```python
from build123d import *

# Parameters (mm, degrees)
SKETCH2_R           = 1.6
BOSS_EXTRUDE1_DEPTH = 4
CUT_EXTRUDE1_DEPTH  = 2
CUT_EXTRUDE2_DEPTH  = 1.5
SKETCH5_R           = 1.5
CUT_EXTRUDE3_DEPTH  = 52.039200621
BOSS_EXTRUDE2_START = 1.5
SKETCH6_R           = 4
SKETCH6_R_2         = 1.5
BOSS_EXTRUDE2_DEPTH = 1.5
CIRPATTERN1_COUNT   = 4
FILLET1_R           = 1
FILLET2_R           = 30


with BuildPart() as part:
    # Sketch2 → Boss-Extrude1 (new body)
    with BuildSketch(Plane(origin=(0, 0, 0), x_dir=(1, 0, 0), z_dir=(0, 1, 0))):
        Polygon((-12.5, 35), (12.5, 35), (23.334523779, 36.062445841), (36.062445841, 23.334523779), (35, 12.5), (35, -12.5), (36.062445841, -23.334523779), (23.334523779, -36.062445841), (12.5, -35), (-12.5, -35), (-23.334523779, -36.062445841), (-36.062445841, -23.334523779), (-35, -12.5), (-35, 12.5), (-36.062445841, 23.334523779), (-23.334523779, 36.062445841), align=None)
        with Locations(Location((22.627416998, 31.112698372, 0), (0, 0, 270))):
            Circle(SKETCH2_R, mode=Mode.SUBTRACT)
        with Locations(Location((31.112698372, 22.627416998, 0), (0, 0, 270))):
            Circle(SKETCH2_R, mode=Mode.SUBTRACT)
        with Locations(Location((22.627416998, -31.112698372, 0), (0, 0, 270))):
            Circle(SKETCH2_R, mode=Mode.SUBTRACT)
        with Locations(Location((31.112698372, -22.627416998, 0), (0, 0, 270))):
            Circle(SKETCH2_R, mode=Mode.SUBTRACT)
        with Locations(Location((-31.112698372, -22.627416998, 0), (0, 0, 270))):
            Circle(SKETCH2_R, mode=Mode.SUBTRACT)
        with Locations(Location((-22.627416998, -31.112698372, 0), (0, 0, 270))):
            Circle(SKETCH2_R, mode=Mode.SUBTRACT)
        with Locations(Location((-22.627416998, 31.112698372, 0), (0, 0, 270))):
            Circle(SKETCH2_R, mode=Mode.SUBTRACT)
        with Locations(Location((-31.112698372, 22.627416998, 0), (0, 0, 270))):
            Circle(SKETCH2_R, mode=Mode.SUBTRACT)
    extrude(amount=BOSS_EXTRUDE1_DEPTH)

    # Sketch3 → Cut-Extrude1 (cut)
    with BuildSketch(Plane(origin=(0, 4, 0), x_dir=(1, 0, 0), z_dir=(0, 1, 0))):
        Polygon((-17.669047558, 29), (17.669047558, 29), (29, 17.669047558), (29, -17.669047558), (17.669047558, -29), (-17.669047558, -29), (-29, -17.669047558), (-29, 17.669047558), align=None)
    extrude(amount=-CUT_EXTRUDE1_DEPTH, mode=Mode.SUBTRACT)

    # Sketch4 → Cut-Extrude2 (cut)
    with BuildSketch(Plane(origin=(0, 2, 0), x_dir=(1, 0, 0), z_dir=(0, 1, 0))):
        with BuildLine():
            Line((-29, 11.263085893), (-29, -11.263085893))
            ThreePointArc((-29, -11.263085893), (-27.272329864, -13.979918004), (-24.079215521, -13.567556979))
            Line((-24.079215521, -13.567556979), (-16.079215521, -6.899529803))
            ThreePointArc((-16.079215521, -6.899529803), (-15.283167889, -5.867388581), (-15, -4.595058717))
            Line((-15, -4.595058717), (-15, 4.595058717))
            ThreePointArc((-15, 4.595058717), (-15.283167889, 5.867388581), (-16.079215521, 6.899529803))
            Line((-16.079215521, 6.899529803), (-24.079215521, 13.567556979))
            ThreePointArc((-24.079215521, 13.567556979), (-27.272329864, 13.979918004), (-29, 11.263085893))
        make_face()
        with BuildLine():
            Line((11.263085893, 29), (-11.263085893, 29))
            ThreePointArc((-11.263085893, 29), (-13.979918004, 27.272329864), (-13.567556979, 24.079215521))
            Line((-13.567556979, 24.079215521), (-6.899529803, 16.079215521))
            ThreePointArc((-6.899529803, 16.079215521), (-5.867388581, 15.283167889), (-4.595058717, 15))
            Line((-4.595058717, 15), (4.595058717, 15))
            ThreePointArc((4.595058717, 15), (5.867388581, 15.283167889), (6.899529803, 16.079215521))
            Line((6.899529803, 16.079215521), (13.567556979, 24.079215521))
            ThreePointArc((13.567556979, 24.079215521), (13.979918004, 27.272329864), (11.263085893, 29))
        make_face()
        with BuildLine():
            Line((29, -11.263085893), (29, 11.263085893))
            ThreePointArc((29, 11.263085893), (27.272329864, 13.979918004), (24.079215521, 13.567556979))
            Line((24.079215521, 13.567556979), (16.079215521, 6.899529803))
            ThreePointArc((16.079215521, 6.899529803), (15.283167889, 5.867388581), (15, 4.595058717))
            Line((15, 4.595058717), (15, -4.595058717))
            ThreePointArc((15, -4.595058717), (15.283167889, -5.867388581), (16.079215521, -6.899529803))
            Line((16.079215521, -6.899529803), (24.079215521, -13.567556979))
            ThreePointArc((24.079215521, -13.567556979), (27.272329864, -13.979918004), (29, -11.263085893))
        make_face()
        with BuildLine():
            Line((-11.263085893, -29), (11.263085893, -29))
            ThreePointArc((11.263085893, -29), (13.979918004, -27.272329864), (13.567556979, -24.079215521))
            Line((13.567556979, -24.079215521), (6.899529803, -16.079215521))
            ThreePointArc((6.899529803, -16.079215521), (5.867388581, -15.283167889), (4.595058717, -15))
            Line((4.595058717, -15), (-4.595058717, -15))
            ThreePointArc((-4.595058717, -15), (-5.867388581, -15.283167889), (-6.899529803, -16.079215521))
            Line((-6.899529803, -16.079215521), (-13.567556979, -24.079215521))
            ThreePointArc((-13.567556979, -24.079215521), (-13.979918004, -27.272329864), (-11.263085893, -29))
        make_face()
    extrude(amount=-CUT_EXTRUDE2_DEPTH, mode=Mode.SUBTRACT)

    # Sketch5 → Cut-Extrude3 (cut, through all)
    with BuildSketch(Plane(origin=(0, 2, 0), x_dir=(1, 0, 0), z_dir=(0, 1, 0))):
        with Locations(Location((13.22775948, 15.25, 0), (0, 0, 270))):
            Circle(SKETCH5_R)
    cut_extrude3 = extrude(amount=-CUT_EXTRUDE3_DEPTH, mode=Mode.SUBTRACT)

    # Sketch6 → Boss-Extrude2 (add)
    with BuildSketch(Plane(origin=(0, 2, 0), x_dir=(1, 0, 0), z_dir=(0, 1, 0)).offset(BOSS_EXTRUDE2_START)):
        with Locations(Location((13.22775948, 15.25, 0), (0, 0, 90))):
            Circle(SKETCH6_R)
        with Locations(Location((13.22775948, 15.25, 0), (0, 0, 270))):
            Circle(SKETCH6_R_2, mode=Mode.SUBTRACT)
    boss_extrude2 = extrude(amount=-BOSS_EXTRUDE2_DEPTH)

    # CirPattern1: Cut-Extrude3, Boss-Extrude2 ×4 about axis
    cirpattern1_axis = Axis((0, 0, 0), (0, 1, 0))
    add([cut_extrude3.rotate(cirpattern1_axis, i * 360 / CIRPATTERN1_COUNT) for i in range(1, CIRPATTERN1_COUNT)], mode=Mode.SUBTRACT)
    add([boss_extrude2.rotate(cirpattern1_axis, i * 360 / CIRPATTERN1_COUNT) for i in range(1, CIRPATTERN1_COUNT)])

    # Fillet1
    fillet1_edges = [part.edges().sort_by_distance(p)[0] for p in [
        (13.22775948, 2, -11.25),
        (-11.25, 2, -13.22775948),
        (-13.22775948, 2, 11.25),
        (11.25, 2, 13.22775948),
    ]]
    fillet(fillet1_edges, radius=FILLET1_R)

    # Fillet2
    # the kernel refuses this fillet: 30 mm, written as the material it adds along each edge
    with BuildSketch(Plane(origin=(-12.5, 0, -35), x_dir=(1, 0, 0), z_dir=(0, 1, 0)), Plane(origin=(-12.5, 0, 35), x_dir=(-0.9952264052892463, 0, 0.09759304388656388), z_dir=(0, 1, 0)), Plane(origin=(-35, 0, 12.5), x_dir=(0, 0, -1), z_dir=(0, 1, 0)), Plane(origin=(-35, 0, -12.5), x_dir=(-0.09759304388655968, 0, -0.9952264052892468), z_dir=(0, 1, 0))) as fillet2_piece_1:
        with BuildLine():
            CenterArc((FILLET2_R * 0.0489132680018, FILLET2_R), FILLET2_R, 264.399415997, 5.600584003)
            Line((-FILLET2_R * 0.0486797758844, FILLET2_R * 0.00477359471072), (0, 0))
            Line((0, 0), (FILLET2_R * 0.0489132680018, 0))
        make_face()
    extrude(amount=4)
    with BuildSketch(Plane(origin=(12.5, 0, -35), x_dir=(-1, 0, 0), z_dir=(0, 1, 0)), Plane(origin=(35, 0, -12.5), x_dir=(0.09759304388620155, 0, -0.9952264052892819), z_dir=(0, 1, 0)), Plane(origin=(35, 0, 12.5), x_dir=(0, 0, -1), z_dir=(0, 1, 0)), Plane(origin=(12.5, 0, 35), x_dir=(0.9952264052892817, 0, 0.09759304388620309), z_dir=(0, 1, 0))) as fillet2_piece_2:
        with BuildLine():
            CenterArc((FILLET2_R * 0.048913268002, -FILLET2_R), FILLET2_R, 90, 5.600584003)
            Line((-FILLET2_R * 0.0486797758846, -FILLET2_R * 0.00477359471075), (0, 0))
            Line((0, 0), (FILLET2_R * 0.048913268002, 0))
        make_face()
    extrude(amount=4)


solid = part.part
```
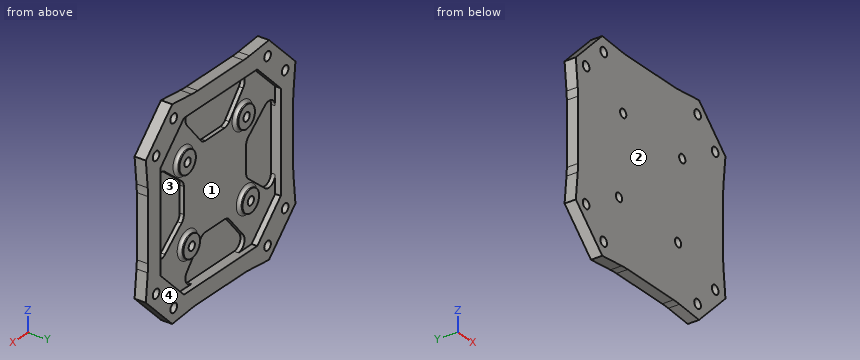
For this review, take the finished solid that the model builds, in its own axes (mm). Face numbers are marked on the shaded views. A direction names the side the tool comes from. Give positions to 0.01 mm unless a question says otherwise; leave off trailing zeros. Write each loop counter-clockwise with the first axis right and the second up, starting at its lowest first coordinate (ties: lowest second). Pieces come first, ordered by that corner, then holes. Notation, with made-up numbers: M -19,-10 L 5,-10 A19 cw 5,-1 Z; hole C 17.25,40 d4. An arc over 180 degrees is marked long. One line per item, written item: value.
1) For the marked faces 3 and 4, list the 3-axis set-ups (+Z, -Z, +X, -X, +Y, -Y) from which the entire face can be reached by the end or side of a thin tool; tool diameter is ignored.
Results are:
face 3: +Y
face 4: +Z, -Z, +X, -X, +Y
2) Take a section at A-A, the plane x = -1. Write out the cut boundary in (y, z), then the cut area to 3 significant figures.
Results are:
outline: M 0,-35 L 4,-35 L 4,-29 L 0.5,-29 L 0.5,-15 L 2,-15 L 2,15 L 0.5,15 L 0.5,29 L 4,29 L 4,35 L 0,35 Z
area: 122 mm²
3) For line 1 (X direction, y = 1.5, z = -1); line 2 (Z direction, x = 10, y = 3.75), list the stretches that pass through material, from the lowest coordinate up. Write a range as from..to.
Results are:
line 1: x = -35..-29, -15..15, 29..35
line 2: z = -35..-29, 29..35
4) Take a section at B-B, the plane z = -26. Write out the cut boundary in (x, y).
Results are:
outline: M -33.4,0 L 33.4,0 L 33.4,4 L 20.67,4 L 20.67,2 L 14.26,2 L 14.26,0.5 L -14.26,0.5 L -14.26,2 L -20.67,2 L -20.67,4 L -33.4,4 Z
5) The part is to be moulded in two halves that separate along X. For the marked faces 1 and 2, say which applies: +X half, -X half, draft (parallel to the pull), parting line (faces both ways), or undercut.
Results are:
face 1: undercut
face 2: draft
6) For P1, Ø1.5, axis at y = 2, z = 11.5, coming from the +X side; P2, Ø1.2, axis at x = -2, y = 1, coming from the -Z side; P3, Ø1.2, axis at y = 1.5, z = 1, coming from the -X side; P4, Ø3, axis at x = -0.5, z = -25.5, coming from the -Y side, all flat-tipped, find the tip position at first contact; note any pin that passes through.
Results are:
P1: stops at x = 35.02
P2: stops at z = -35
P3: stops at x = -35
P4: stops at y = 0
